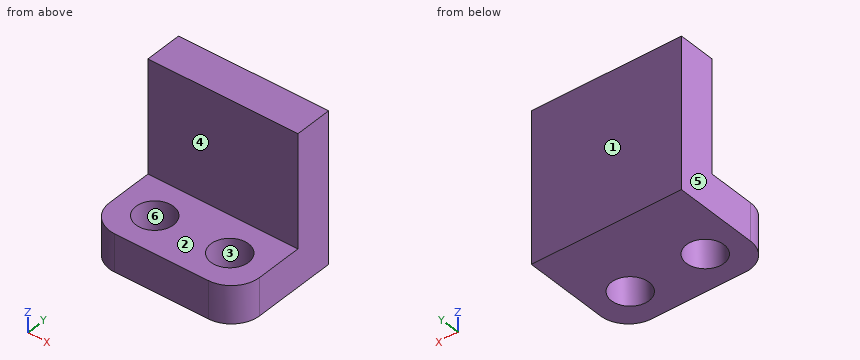
from build123d import *

# Parameters (mm, degrees)
F0_W     = 20.32
F0_H     = 5.08
F1_DEPTH = 15.24
F2_R     = 3.81
F4_D     = 5.08
F5_W     = 20.32
F5_H     = 5.08
F6_DEPTH = 15.24


with BuildPart() as f1:
    # F0 (on Front) → F1 (new body)
    with BuildSketch(Plane.XZ):
        with Locations((10.16, 2.54)):
            Rectangle(F0_W, F0_H)
    extrude(amount=F1_DEPTH)

    # F2
    f2_edges = [f1.edges().sort_by_distance(p)[0] for p in [
        (20.32, -15.24, 2.54),
        (0, -15.24, 2.54),
    ]]
    fillet(f2_edges, radius=F2_R)

    # F4 (through all)
    with Locations(Plane.XY.offset(5.08)):
        with Locations((5.08, -10.16), (15.24, -10.16)):
            Hole(F4_D / 2)

    # F5 (on face) → F6 (join)
    with BuildSketch(Plane.XY.offset(5.08)):
        with Locations((10.16, -2.54)):
            Rectangle(F5_W, F5_H)
    extrude(amount=F6_DEPTH)


solid = f1.part
Design review of the part built by this model. Coordinates are the model's own, in mm. Face numbers are marked on the shaded views. A direction names the side the tool comes from. Give positions to 0.01 mm unless a question says otherwise; leave off trailing zeros. Loops run counter-clockwise (first coordinate to the right, second up) from the corner with the lowest first, then second, coordinate; pieces in that order, holes last. Notation, with made-up numbers: M -5,-1.5 L 26,-1.5 A25 ccw 26,11.5 Z; hole C -25,6 d1. An arc over 180 degrees is marked long. Answer as a JSON object with one key per item and string values.
Item 1: We need section A-A (x = 15.24). State the section outline as (y, z) points, and give its area (3 significant figures).
Output values:
{"outline": "M -15.24,0 L -12.7,0 L -12.7,5.08 L -15.24,5.08 Z; M -7.62,0 L 0,0 L 0,20.32 L -5.08,20.32 L -5.08,5.08 L -7.62,5.08 Z", "area": "129 mm2"}
Item 2: We need section B-B (y = -10.16). State the section outline as (x, z) points, and give its area (3 significant figures).
Output values:
{"outline": "M 0,0 L 2.54,0 L 2.54,5.08 L 0,5.08 Z; M 7.62,0 L 12.7,0 L 12.7,5.08 L 7.62,5.08 Z; M 17.78,0 L 20.32,0 L 20.32,5.08 L 17.78,5.08 Z", "area": "51.6 mm2"}
Item 3: Mouldability with a two-part tool opening along Y and no side actions: class the marked faces 3, 4, 5 and 6 as pulls with the +Y half, pulls with the -Y half, needs draft (parallel to the pull), parting line crosses it, or undercut.
Output values:
{"face 3": "undercut", "face 4": "pulls with the -Y half", "face 5": "needs draft", "face 6": "undercut"}
Item 4: We need section D-D (x = 1.5). State the section outline as (y, z) points.
Output values:
{"outline": "M -14.46,0 L 0,0 L 0,20.32 L -5.08,20.32 L -5.08,5.08 L -14.46,5.08 Z"}
Item 5: We need section C-C (y = -5.75). State the section outline as (x, z) points, and give its area (3 significant figures).
Output values:
{"outline": "M 0,0 L 20.32,0 L 20.32,5.08 L 0,5.08 Z", "area": "103 mm2"}
Item 6: Wall thickness on line 1 along Y through (x, z) = (15.24, 3.35); line 2 along Y through (x, z) = (6.75, 15.25); line 3 along Y through (x, z) = (17.25, 1.75): over which ranges is each line inside the solid? List them lowest first.
Output values:
{"line 1": "y = -15.24 to -12.7, -7.62 to 0", "line 2": "y = -5.08 to 0", "line 3": "y = -15.17 to -11.71, -8.61 to 0"}
Item 7: For P1, Ø1, axis at x = 14, y = -8.5, coming from the +Z side; P2, Ø12, axis at x = 5, z = 14, coming from the -Y side, all flat-tipped, find the tip position at first contact; note any pin that passes through.
Output values:
{"P1": "stops at z = 5.08", "P2": "stops at y = -5.08"}
Item 8: Machinability: for the marked faces 1 and 2, which of the approach directions +Z, -Z, +X, -X, +Y, -Y give a long, thin tool a straight path to every point of the face, cutting with its end or side? Answer none if there is none.
Output values:
{"face 1": "+Z, -Z, +X, -X, +Y", "face 2": "+Z, +X, -X, -Y"}
